Work out the finished part from the listing and answer in its coordinate system (mm). Face numbers are marked on the shaded views. A direction names the side the tool comes from. Coordinates: 2 decimals unless noted, no trailing zeros. Order: outer loops, then holes, each group sorted by start corner. A loop starts at its lowest first (then second) coordinate and runs counter-clockwise, first axis right, second up. Notation, with made-up numbers: M 66,29.5 L 122,29.5 A12 ccw 122,43.5 Z; hole C 43,84.5 d8. An arc over 180 degrees is marked long. Use a Markdown table: item, result.
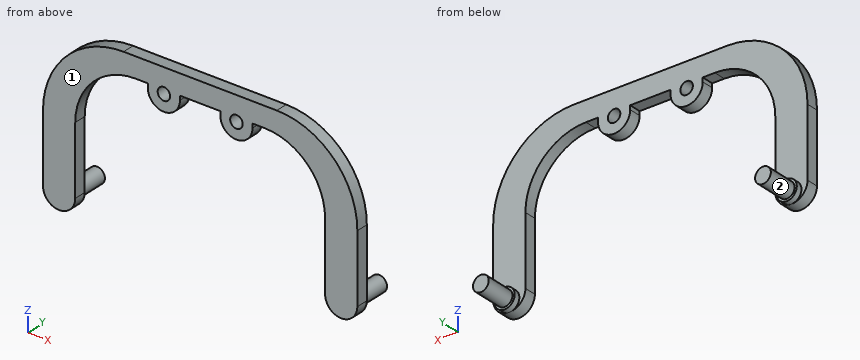
from build123d import *

# Parameters (mm, degrees)
EXTRUDE_1_DEPTH     = 3
SKETCH_2_R          = 1.55
CUT_EXTRUDE_1_DEPTH = 3
SKETCH_3_R          = 1.95
EXTRUDE_2_DEPTH     = 9
FILLET_4_RADIUS     = 4
FILLET_4_LENGTH     = 3
FILLET_5_RADIUS     = 4
FILLET_5_LENGTH     = 3
SKETCH_4_R          = 2.5
EXTRUDE_3_DEPTH     = 1.48
FILLET_6_R          = 15
FILLET_7_R          = 20
CUT_EXTRUDE_2_DEPTH = 55.5068803


with BuildPart() as part:
    # 草图1 → 凸台-拉伸1 (new body)
    with BuildSketch(Plane(origin=(0, 0, 0), x_dir=(1, 0, 0), z_dir=(0, 1, 0))):
        Polygon((-39, 37), (-31, 37), (-31, 0), (-13, 0), (-13, 5), (-5, 5), (-5, 0), (0, 0), (0, -5), (-39, -5), align=None)
    extrude_1 = extrude(amount=EXTRUDE_1_DEPTH)

    # 草图2 → 切除-拉伸1 (cut)
    with BuildSketch(Plane(origin=(0, 3, 0), x_dir=(1, 0, 0), z_dir=(0, 1, 0))):
        with Locations(Location((-9, 1, 0), (0, 0, 270))):
            Circle(SKETCH_2_R)
    cut_extrude_1 = extrude(amount=-CUT_EXTRUDE_1_DEPTH, mode=Mode.SUBTRACT)

    # 草图3 → 凸台-拉伸2 (add)
    with BuildSketch(Plane(origin=(0, 3, 0), x_dir=(1, 0, 0), z_dir=(0, 1, 0))):
        with Locations(Location((-35, 33.5, 0), (0, 0, 90))):
            Circle(SKETCH_3_R)
    extrude_2 = extrude(amount=EXTRUDE_2_DEPTH)

    # 镜向1: 凸台-拉伸1, 切除-拉伸1, 凸台-拉伸2 across plane
    add(extrude_1.mirror(Plane(origin=(0, 3, 0), x_dir=(0, 0, 1), z_dir=(-1, 0, 0))))
    add(cut_extrude_1.mirror(Plane(origin=(0, 3, 0), x_dir=(0, 0, 1), z_dir=(-1, 0, 0))), mode=Mode.SUBTRACT)
    add(extrude_2.mirror(Plane(origin=(0, 3, 0), x_dir=(0, 0, 1), z_dir=(-1, 0, 0))))

    # 圆角4: full round fillet: the end face becomes a half cylinder, R = half its width
    fillet_4_face = Plane((-9, 1.5, -5), x_dir=(0, 1, 0), z_dir=(0, 0, -1))  # on the end face: x along it, z out of the body
    fillet_4_slab = fillet_4_face.offset(-FILLET_4_RADIUS / 2) * Box(FILLET_4_LENGTH, 2 * FILLET_4_RADIUS, FILLET_4_RADIUS, mode=Mode.PRIVATE)  # the body's end, R deep
    fillet_4_round = Plane((-9, 1.5, -1), x_dir=(0, 0, -1), z_dir=(0, 1, 0)) * Cylinder(FILLET_4_RADIUS, FILLET_4_LENGTH, mode=Mode.PRIVATE)  # its axis R under the face
    add(fillet_4_slab - fillet_4_round, mode=Mode.SUBTRACT)

    # 圆角5: full round fillet: the end face becomes a half cylinder, R = half its width
    fillet_5_face = Plane((9, 1.5, -5), x_dir=(0, -1, 0), z_dir=(0, 0, -1))  # on the end face: x along it, z out of the body
    fillet_5_slab = fillet_5_face.offset(-FILLET_5_RADIUS / 2) * Box(FILLET_5_LENGTH, 2 * FILLET_5_RADIUS, FILLET_5_RADIUS, mode=Mode.PRIVATE)  # the body's end, R deep
    fillet_5_round = Plane((9, 1.5, -1), x_dir=(0, 0, -1), z_dir=(0, -1, 0)) * Cylinder(FILLET_5_RADIUS, FILLET_5_LENGTH, mode=Mode.PRIVATE)  # its axis R under the face
    add(fillet_5_slab - fillet_5_round, mode=Mode.SUBTRACT)

    # 草图4 → 凸台-拉伸3 (add)
    with BuildSketch(Plane(origin=(0, 3, 0), x_dir=(1, 0, 0), z_dir=(0, 1, 0))):
        with Locations(Location((-35, 33.5, 0), (0, 0, 90))):
            Circle(SKETCH_4_R)
    extrude_3 = extrude(amount=EXTRUDE_3_DEPTH)

    # 镜向2: 凸台-拉伸3 across plane
    add(extrude_3.mirror(Plane(origin=(0, 0, 0), x_dir=(0, 0, 1), z_dir=(1, 0, 0))))

    # 圆角6
    fillet_6_edges = [part.edges().sort_by_distance(p)[0] for p in [
        (-31, 1.5, 0),
        (31, 1.5, 0),
    ]]
    fillet(fillet_6_edges, radius=FILLET_6_R)

    # 圆角7
    fillet_7_edges = [part.edges().sort_by_distance(p)[0] for p in [
        (-39, 1.5, 5),
        (39, 1.5, 5),
    ]]
    fillet(fillet_7_edges, radius=FILLET_7_R)

    # 草图5 → 切除-拉伸2 (cut, through all)
    with BuildSketch(Plane(origin=(0, 3, 0), x_dir=(1, 0, 0), z_dir=(0, 1, 0))):
        with BuildLine():
            Line((-39, 32), (-39, 37))
            Line((-39, 37), (-31, 37))
            Line((-31, 37), (-31, 32))
            ThreePointArc((-31, 32), (-35, 36), (-39, 32))
        make_face()
    cut_extrude_2 = extrude(amount=-CUT_EXTRUDE_2_DEPTH, mode=Mode.SUBTRACT)

    # 镜向3: 切除-拉伸2 across plane
    add(cut_extrude_2.mirror(Plane(origin=(0, 0, 0), x_dir=(0, 0, 1), z_dir=(1, 0, 0))), mode=Mode.SUBTRACT)


solid = part.part
(1) A cutting plane is placed at C-C (y = 1). Determine the outline of the cut face in (x, z), then the cut area to 3 significant figures.
Conclusion:
| item | result |
|---|---|
| outline | M -39,-32 A4 ccw -31,-32 L -31,-15 A15 cw -16,0 L -13,0 L -13,-1 A4 ccw -5,-1 L -5,0 L 5,0 L 5,-1 A4 ccw 13,-1 L 13,0 L 16,0 A15 cw 31,-15 L 31,-32 A4 ccw 39,-32 L 39,-15 A20 ccw 19,5 L -19,5 A20 ccw -39,-15 Z; hole C -9,-1 d3.1; hole C 9,-1 d3.1 |
| area | 928 mm2 |
(2) A cutting plane is placed at A-A (x = 9). Determine the outline of the cut face in (y, z).
Conclusion:
| item | result |
|---|---|
| outline | M 0,-5 L 3,-5 L 3,-2.55 L 0,-2.55 Z; M 0,0.55 L 3,0.55 L 3,5 L 0,5 Z |
(3) Straight lines are drawn through the part: L1, parallel to X at y = 1.75, z = -28.5; L2, parallel to Y at x = 34, z = -26; L3, parallel to Z at x = -15.5, y = 1.75. For each, find the intervals that lie inside material, in ascending order.
Conclusion:
| item | result |
|---|---|
| L1 | -39 to -31, 31 to 39 |
| L2 | 0 to 3 |
| L3 | 0 to 5 |
(4) Given P1, Ø4, axis at x = 17, y = 2, coming from the -Z side; P2, Ø1.1, axis at y = 1.5, z = -0.5, coming from the -X side; P3, Ø0.9, axis at x = -2.5, y = 1.5, coming from the -Z side; P4, Ø2.5, axis at x = 9, z = -1, coming from the -Y side, each flat-ended and moving along its own axis, determine where each tip first touches the part or whether it passes through.
Conclusion:
| item | result |
|---|---|
| P1 | z = -0.3 |
| P2 | x = -33.33 |
| P3 | z = 0 |
| P4 | through |
(5) A cutting plane is placed at B-B (z = -25). Determine the outline of the cut face in (x, y).
Conclusion:
| item | result |
|---|---|
| outline | M -39,0 L -31,0 L -31,3 L -39,3 Z; M 31,0 L 39,0 L 39,3 L 31,3 Z |
(6) A cutting plane is placed at D-D (y = 6.25). Determine the outline of the cut face in (x, z).
Conclusion:
| item | result |
|---|---|
| outline | C -35,-33.5 d3.9; C 35,-33.5 d3.9 |
(7) Which of the six approach directions +Z, -Z, +X, -X, +Y, -Y give full straight-line access (tool end or side, diameter ignored) to the marked faces 1 and 2?
Conclusion:
| item | result |
|---|---|
| face 1 | +Z, -Z, +X, -X, -Y |
| face 2 | +Y |
